```python
from build123d import *

# Parameters (mm, degrees)
BOSS_EXTRUDE1_DEPTH = 50.8
SKETCH2_W           = 12.7
SKETCH2_H           = 3.175
BOSS_EXTRUDE2_DEPTH = 2.9972
SKETCH3_R           = 1.499997
CUT_EXTRUDE1_DEPTH  = 71.299547696
FILLET1_R           = 25.4


with BuildPart() as part:
    # Sketch1 → Boss-Extrude1 (new body)
    with BuildSketch(Plane(origin=(0, 0, 0), x_dir=(0, 0, -1), z_dir=(1, 0, 0))):
        Polygon((0, 0), (-42.8625, 0), (-42.8625, 4.7625), (-4.7625, 4.7625), (-4.7625, 30.1625), (0, 30.1625), align=None)
    extrude(amount=BOSS_EXTRUDE1_DEPTH)

    # Sketch2 → Boss-Extrude2 (add)
    with BuildSketch(Plane(origin=(0, 4.7625, 0), x_dir=(1, 0, 0), z_dir=(0, 1, 0))):
        with Locations((25.4, -19.05)):
            Rectangle(SKETCH2_W, SKETCH2_H)
    extrude(amount=BOSS_EXTRUDE2_DEPTH)

    # Sketch3 → Cut-Extrude1 (cut, through all)
    with BuildSketch(Plane.XY.offset(4.7625)):
        with Locations((25.4, 23.8125)):
            Circle(SKETCH3_R)
    extrude(amount=-CUT_EXTRUDE1_DEPTH, mode=Mode.SUBTRACT)

    # Fillet1
    fillet1_edges = [part.edges().sort_by_distance(p)[0] for p in [
        (0, 30.1625, 2.38125),
        (50.8, 30.1625, 2.38125),
    ]]
    fillet(fillet1_edges, radius=FILLET1_R - 0.0001)  # a hair under: the kernel refuses the full size


solid = part.part
```
Geometry check sheet. Reference: the model listing, model coordinates, mm. A direction names the side the tool comes from. Give positions to 0.01 mm unless a question says otherwise; leave off trailing zeros. Order: outer loops, then holes, each group sorted by start corner. A loop starts at its lowest first (then second) coordinate and runs counter-clockwise, first axis right, second up. Notation, with made-up numbers: (23, -38.75) -> (79, -38.75) arc R17 ccw to (79, -30.75) -> close; hole circle Ø9 at (56.5, 1.5). An arc over 180 degrees is marked (long way). Write each question's results on one line, items separated by ' | '. Start each with the question number.
(1) Sectioned sample at A-A (x = 37). Enter the section's corners in (y, z).
(2) Access from +Z, -Z, +X, -X, +Y, -Y to the whole of each face (thin tool, end or side, straight path). Record for faces 1 (the face through (31.75, 6, 19)), 2 (the face through (19.05, 6, 19)), 3 (the face through (25, 7.76, 19)).
(3) Gauge pin test, flat ends, axial feed: P1, Ø12.5, axis at x = 34.5, y = 15, coming from the +Z side; P2, Ø10, axis at x = 39.5, z = 37.5, coming from the +Y side; P3, Ø2.5, axis at y = 7, z = 19, coming from the +X side. Record the tip position at first contact, or that the pin passes through.
(4) Sectioned sample at C-C (y = 18.5). Enter the section's corners in (x, z), plus the area to 3 significant figures.
(5) Scan lines: line 1 (Y direction, x = 25.4, z = 3.5); line 2 (Y direction, x = 21, z = 21). Record each from-to range of solid material in increasing order.
(6) Mould release check, pull along Z, two halves, no side actions. Record for faces 4 (the face through (50.8, 2, 21)), 5 (the face through (25, 6, 20.638)), 6 (the face through (25, 6, 17.463)): pulls with the +Z half, pulls with the -Z half, needs draft (parallel to the pull), parting line crosses it, or undercut.
(7) Sectioned sample at D-D (x = 31). Enter the section's corners in (y, z), plus the area to 3 significant figures.
(8) Sectioned sample at B-B (z = 10). Enter the section's corners in (x, y).
Answer below:
1) outline: (0, 0) -> (27.36, 0) -> (27.36, 4.76) -> (4.76, 4.76) -> (4.76, 42.86) -> (0, 42.86) -> close
2) face 1: +Z, +X, +Y | face 2: +Z, -X, +Y | face 3: +Z, +X, -X, +Y
3) P1: z = 4.76 | P2: y = 4.76 | P3: x = 31.75
4) outline: (4.04, 0) -> (46.76, 0) -> (46.76, 4.76) -> (4.04, 4.76) -> close | area: 203 mm2
5) line 1: 0 to 22.31, 25.31 to 30.16 | line 2: 0 to 4.76
6) face 4: needs draft | face 5: pulls with the +Z half | face 6: undercut
7) outline: (0, 0) -> (29.54, 0) -> (29.54, 4.76) -> (4.76, 4.76) -> (4.76, 17.46) -> (7.76, 17.46) -> (7.76, 20.64) -> (4.76, 20.64) -> (4.76, 42.86) -> (0, 42.86) -> close | area: 332 mm2
8) outline: (0, 0) -> (50.8, 0) -> (50.8, 4.76) -> (0, 4.76) -> close
